```python
from build123d import *

# Parameters (mm, degrees)
SKETCH1_W           = 29
SKETCH1_H           = 71
BOSS_EXTRUDE1_DEPTH = 1.5
SKETCH2_W           = 29
SKETCH2_H           = 71
SKETCH2_W_2         = 26
SKETCH2_H_2         = 68
BOSS_EXTRUDE2_DEPTH = 10
SKETCH3_R           = 3.5
CUT_EXTRUDE1_DEPTH  = 9


with BuildPart() as part:
    # Sketch1 → Boss-Extrude1 (new body)
    with BuildSketch(Plane(origin=(0, 0, 0), x_dir=(1, 0, 0), z_dir=(0, 1, 0))):
        with Locations((14.5, 35.5)):
            Rectangle(SKETCH1_W, SKETCH1_H)
    extrude(amount=BOSS_EXTRUDE1_DEPTH)

    # Sketch2 → Boss-Extrude2 (add)
    with BuildSketch(Plane(origin=(0, 1.5, 0), x_dir=(1, 0, 0), z_dir=(0, 1, 0))):
        with Locations((14.5, 35.5)):
            Rectangle(SKETCH2_W, SKETCH2_H)
        with Locations((14.5, 35.5)):
            Rectangle(SKETCH2_W_2, SKETCH2_H_2, mode=Mode.SUBTRACT)
    extrude(amount=BOSS_EXTRUDE2_DEPTH)

    # Sketch3 → Cut-Extrude1 (cut)
    with BuildSketch(Plane(origin=(0, 0, -1.5), x_dir=(-1, 0, 0), z_dir=(0, 0, -1))):
        with Locations((-14.5, 6.5)):
            Circle(SKETCH3_R)
    extrude(amount=-CUT_EXTRUDE1_DEPTH, mode=Mode.SUBTRACT)


solid = part.part
```
For this review, take the finished solid that the model builds, in its own axes (mm). A direction names the side the tool comes from. Coordinates: 2 decimals unless noted, no trailing zeros. Loops run counter-clockwise (first coordinate to the right, second up) from the corner with the lowest first, then second, coordinate; pieces in that order, holes last. Notation, with made-up numbers: (21.25, 63) - (36.25, 63) arc R33 cw to (36.25, 97) - close; hole circle Ø3 at (56, 53.25). An arc over 180 degrees is marked (long way). Use one line per item in the form item = value. Start each with the question number.
1) Take a section at B-B (x = 4.5). State the section outline as (y, z) points.
2) For faces 5 (the face through (0.5, 11.5, -35.7)), 6 (the face through (14, 6, -69.5)), list the 3-axis set-ups (+Z, -Z, +X, -X, +Y, -Y) from which the entire face can be reached by the end or side of a thin tool; tool diameter is ignored.
3) Take a section at D-D (x = 14.5). State the section outline as (y, z) points, plus the area to 3 significant figures.
4) To check wall thickness, follow probe 1 along Y at (x, z) = (14.5, -0.95); probe 2 along X at (y, z) = (6.25, -33); probe 3 along Z at (x, y) = (26.25, 8). State the ranges of each line that lie inside material, in increasing order. Write a range as from..to.
5) Take a section at C-C (z = -52). State the section outline as (x, y) points, plus the area to 3 significant figures.
6) Take a section at A-A (y = 6.5). State the section outline as (x, z) points, plus the area to 4 significant figures.
7) For pin 1 (8 mm diameter, centred on x = 19, z = -24.5, fed in from +Y), flat-tipped, find the tip position at first contact; note if it passes through.
8) Draft analysis for pull direction Z (two halves, no side actions). For faces 1 (the face through (27.5, 6, -35)), 2 (the face through (11.267, 5.159, -0.76)), 3 (the face through (11, 4, 0)), 4 (the face through (14, 6, -71)), state which applies: released by +Z, released by -Z, zero draft, split by the parting line, or undercut.
From the geometry:
q1.outline = (0, -71) - (11.5, -71) - (11.5, -69.5) - (1.5, -69.5) - (1.5, -1.5) - (11.5, -1.5) - (11.5, 0) - (0, 0) - close
q2.face_5 = +Z, -Z, +X, -X, +Y
q2.face_6 = +Y
q3.outline = (0, -71) - (11.5, -71) - (11.5, -69.5) - (1.5, -69.5) - (1.5, -1.5) - (3, -1.5) - (3, 0) - (0, 0) - close; (10, -1.5) - (11.5, -1.5) - (11.5, 0) - (10, 0) - close
q3.area = 126 mm2
q4.probe_1 = 0..3, 10..11.5
q4.probe_2 = 0..1.5, 27.5..29
q4.probe_3 = -71..-69.5, -1.5..0
q5.outline = (0, 0) - (29, 0) - (29, 11.5) - (27.5, 11.5) - (27.5, 1.5) - (1.5, 1.5) - (1.5, 11.5) - (0, 11.5) - close
q5.area = 73.5 mm2
q6.outline = (0, -71) - (29, -71) - (29, 0) - (18, 0) - (18, -1.5) - (27.5, -1.5) - (27.5, -69.5) - (1.5, -69.5) - (1.5, -1.5) - (11, -1.5) - (11, 0) - (0, 0) - close
q6.area = 280.5 mm2
q7.pin_1 = 1.5
q8.face_1 = undercut
q8.face_2 = zero draft
q8.face_3 = released by +Z
q8.face_4 = released by -Z
